Verification items for the finished model (mm, model axes). A direction names the side the tool comes from. Round coordinates to 2 decimals unless told otherwise and drop trailing zeros. Order: outer loops, then holes, each group sorted by start corner. A loop starts at its lowest first (then second) coordinate and runs counter-clockwise, first axis right, second up. Notation, with made-up numbers: M 17.5,-40 L 42.5,-40 A27 cw 42.5,-20 Z; hole C -13.5,84 d11. An arc over 180 degrees is marked long. Answer as a JSON object with one key per item and string values. Group by question number.
```python
from build123d import *

# Parameters (mm, degrees)
SKETCH_R     = 2.4
PAD_DEPTH    = 5
SKETCH001_R  = 4
POCKET_DEPTH = 3


with BuildPart() as part:
    # Sketch → Pad (new body)
    with BuildSketch(Plane.XY):
        with BuildLine():
            Line((-39, 28), (39, 28))
            ThreePointArc((44, 23), (42.535534, 26.535534), (39, 28))
            Line((44, 23), (44, -23))
            ThreePointArc((39, -28), (42.535534, -26.535534), (44, -23))
            Line((39, -28), (-39, -28))
            ThreePointArc((-44, -23), (-42.535534, -26.535534), (-39, -28))
            Line((-44, -23), (-44, 23))
            ThreePointArc((-39, 28), (-42.535534, 26.535534), (-44, 23))
        make_face()
        with Locations((-38.25, 0)):
            Circle(SKETCH_R, mode=Mode.SUBTRACT)
        with Locations((38.25, 0)):
            Circle(SKETCH_R, mode=Mode.SUBTRACT)
    extrude(amount=PAD_DEPTH)

    # Sketch001 (on Face12 of Pad) → Pocket (cut)
    with BuildSketch(Plane.XY.offset(5)):
        with Locations((-38.25, 0)):
            Circle(SKETCH001_R)
        with Locations((38.25, 0)):
            Circle(SKETCH001_R)
    extrude(amount=-POCKET_DEPTH, mode=Mode.SUBTRACT)


solid = part.part
```
Q1. Cross-section at A-A, the plane z = 3.95. Record the cut outline in (x, y).
Q2. Tool access check on faces 4 (the face through (1, 0, 0)), 5 (the face through (-35.6, 0.1, 2)). Record the directions out of +Z, -Z, +X, -X, +Y, -Y that give a thin tool (end or side, any length) a straight path to the whole face; none if there is none.
Q3. Gauge pin test, flat end, axial feed: pin 1 Ø7.5 at (x, y) = (38.25, 0) entering from +Z. Record the tip position at first contact, or that the pin passes through.
Q4. Cross-section at C-C, the plane x = -37. Record the cut outline in (y, z), then the cut area to 3 significant figures.
Q5. Cross-section at B-B, the plane y = 0. Record the cut outline in (x, z).
Q6. Release check for a two-part mould opening along Y. For faces 1 (the face through (1, 0, 5)), 2 (the face through (43, 26, 2)), 3 (the face through (-40.648, 0.106, 0.986)) record: released by +Y, released by -Y, zero draft, split by the parting line, or undercut.
Q7. Thickness scan on line 1 (X direction, y = 0, z = 0.75); line 2 (Y direction, x = -38.25, z = 3.2); line 3 (Y direction, x = -38.25, z = 1.05). Record the ranges inside material, lowest first. Write a range as from..to.
Conclusion:
{
 "1": {"outline": "M -44,-23 A5 ccw -39,-28 L 39,-28 A5 ccw 44,-23 L 44,23 A5 ccw 39,28 L -39,28 A5 ccw -44,23 Z; hole C -38.25,0 d8; hole C 38.25,0 d8"},
 "2": {"face 4": "-Z, +X, -X, +Y, -Y", "face 5": "+Z"},
 "3": {"pin 1": "z = 2"},
 "4": {"outline": "M -28,0 L -2.05,0 L -2.05,2 L -3.8,2 L -3.8,5 L -28,5 Z; M 2.05,0 L 28,0 L 28,5 L 3.8,5 L 3.8,2 L 2.05,2 Z", "area": "249 mm2"},
 "5": {"outline": "M -44,0 L -40.65,0 L -40.65,2 L -42.25,2 L -42.25,5 L -44,5 Z; M -35.85,0 L 35.85,0 L 35.85,2 L 34.25,2 L 34.25,5 L -34.25,5 L -34.25,2 L -35.85,2 Z; M 40.65,0 L 44,0 L 44,5 L 42.25,5 L 42.25,2 L 40.65,2 Z"},
 "6": {"face 1": "zero draft", "face 2": "released by +Y", "face 3": "undercut"},
 "7": {"line 1": "-44..-40.65, -35.85..35.85, 40.65..44", "line 2": "-28..-4, 4..28", "line 3": "-28..-2.4, 2.4..28"}
}
